Can you work these out from the model? Positions are in its coordinate system, mm. Round coordinates to 2 decimals unless told otherwise and drop trailing zeros. Write each loop counter-clockwise with the first axis right and the second up, starting at its lowest first coordinate (ties: lowest second). Pieces come first, ordered by that corner, then holes. Notation, with made-up numbers: M 21.5,29.5 L 40.5,29.5 A23 ccw 40.5,62.5 Z; hole C 52,39 d3. An arc over 180 degrees is marked long. Answer in a Markdown table with one row per item. Add a question column.
(1) Suppose I cut it at C-C, the plane z = -74. Count the separate pieces of the cut face and the enclosed holes in it, then the cut area to 3 significant figures.
(2) I'm going to push flat-ended pins straight in: pin 1 (22 mm diameter, centred on x = 342.5, y = 112, fed in from +Z); pin 2 (5 mm diameter, centred on x = 236, y = 171.5, fed in from +Z). Where does each tip first touch, or does it pass through?
(3) If I drill on probe 1 along Y at (x, z) = (177.5, -43.5); probe 2 along X at (y, z) = (66.5, -177); probe 3 along Z at (x, y) = (96, 211), over which ranges is the centre line in solid material (lowest first)?
(4) Suppose I cut it at A-A, the plane y = 112.5. Write out the boundary of the cut face in (x, z).
(5) Suppose I cut it at B-B, the plane x = 369. Write out the boundary of the cut face in (y, z), then the cut area to 3 significant figures.
(6) If we mould it in two halves opening along Y, with no side actions, what happens to faces 1 (the face through (138.333, 208, -148)), 2 (the face through (203, -5, -158))? For each: released by +Y, released by -Y, zero draft, split by the parting line, or undercut.
from build123d import *

# Parameters (mm, degrees)
CROQUIS1_W              = 410
CROQUIS1_H              = 260
CROQUIS1_W_2            = 123.333333333
CROQUIS1_H_2            = 73.333333333
CROQUIS1_W_3            = 123.333333334
CROQUIS1_H_3            = 73.333333334
SALIENTE_EXTRUIR3_DEPTH = 300
CROQUIS4_W              = 410
CROQUIS4_H              = 260
SALIENTE_EXTRUIR4_DEPTH = 20


with BuildPart() as part:
    # Croquis1 → Saliente-Extruir3 (new body)
    with BuildSketch(Plane.XY):
        with Locations((200, 125)):
            Rectangle(CROQUIS1_W, CROQUIS1_H)
        with Locations((66.666666667, 41.666666666)):
            Rectangle(CROQUIS1_W_2, CROQUIS1_H_2, mode=Mode.SUBTRACT)
        with Locations((200, 41.666666666)):
            Rectangle(CROQUIS1_W_3, CROQUIS1_H_2, mode=Mode.SUBTRACT)
        with Locations((333.333333334, 125)):
            Rectangle(CROQUIS1_W_2, CROQUIS1_H_3, mode=Mode.SUBTRACT)
        with Locations((333.333333334, 41.666666666)):
            Rectangle(CROQUIS1_W_2, CROQUIS1_H_2, mode=Mode.SUBTRACT)
        with Locations((66.666666667, 125)):
            Rectangle(CROQUIS1_W_2, CROQUIS1_H_3, mode=Mode.SUBTRACT)
        with Locations((66.666666667, 208.333333334)):
            Rectangle(CROQUIS1_W_2, CROQUIS1_H_2, mode=Mode.SUBTRACT)
        with Locations((200, 125)):
            Rectangle(CROQUIS1_W_3, CROQUIS1_H_3, mode=Mode.SUBTRACT)
        with Locations((200, 208.333333334)):
            Rectangle(CROQUIS1_W_3, CROQUIS1_H_2, mode=Mode.SUBTRACT)
        with Locations((333.333333334, 208.333333334)):
            Rectangle(CROQUIS1_W_2, CROQUIS1_H_2, mode=Mode.SUBTRACT)
    extrude(amount=-SALIENTE_EXTRUIR3_DEPTH)

    # Croquis4 → Saliente-Extruir4 (add)
    with BuildSketch(Plane(origin=(0, 0, -300), x_dir=(-1, 0, 0), z_dir=(0, 0, -1))):
        with Locations((-200, 125)):
            Rectangle(CROQUIS4_W, CROQUIS4_H)
    extrude(amount=SALIENTE_EXTRUIR4_DEPTH)


solid = part.part
Calculated:
| question | item | result |
|---|---|---|
| 1 | separate pieces | 1 |
| 1 | enclosed holes | 9 |
| 1 | area | 25,200 mm² |
| 2 | pin 1 | z = -300 |
| 2 | pin 2 | z = 0 |
| 3 | probe 1 | -5 to 5, 78.33 to 88.33, 161.67 to 171.67, 245 to 255 |
| 3 | probe 2 | -5 to 5, 128.33 to 138.33, 261.67 to 271.67, 395 to 405 |
| 3 | probe 3 | -320 to -300 |
| 4 | outline | M -5,-320 L 405,-320 L 405,0 L 395,0 L 395,-300 L 271.67,-300 L 271.67,0 L 261.67,0 L 261.67,-300 L 138.33,-300 L 138.33,0 L 128.33,0 L 128.33,-300 L 5,-300 L 5,0 L -5,0 Z |
| 5 | outline | M -5,-320 L 255,-320 L 255,0 L 245,0 L 245,-300 L 171.67,-300 L 171.67,0 L 161.67,0 L 161.67,-300 L 88.33,-300 L 88.33,0 L 78.33,0 L 78.33,-300 L 5,-300 L 5,0 L -5,0 Z |
| 5 | area | 17,200 mm² |
| 6 | face 1 | undercut |
| 6 | face 2 | released by -Y |
